```python
from build123d import *

# Parameters (mm, degrees)
F0_W            = 61.5
F0_H            = 60.53
F1_DEPTH        = 4.38
F3_DEPTH        = 31.34
F4_W            = 5.65
F4_H            = 8.3
F4_W_2          = 8.3
F4_H_2          = 5.65
F5_DEPTH        = 35.72
F7_DEPTH        = 35.72
F9_DEPTH        = 35.72
F11_D           = 3.5
F11_CSINK_D     = 10
F11_CSINK_ANGLE = 90
F13_D           = 3.5
F13_CSINK_D     = 10
F13_CSINK_ANGLE = 90
F15_D           = 3.5
F15_CSINK_D     = 10
F15_CSINK_ANGLE = 90
F17_D           = 3.5
F17_CSINK_D     = 10
F17_CSINK_ANGLE = 90


with BuildPart() as f1:
    # F0 (on Top) → F1 (new body)
    with BuildSketch(Plane.XY):
        with Locations((-10.297848, 8.882269)):
            Rectangle(F0_W, F0_H)
    extrude(amount=F1_DEPTH)

    # F2 (on face) → F3 (join)
    with BuildSketch(Plane.XY.offset(4.38)):
        Polygon((-41.047848, 39.147269), (-41.047848, -21.382731), (-35.397848, -21.382731), (-35.397848, 33.497269), (20.452152, 33.497269), (20.452152, 39.147269), (-35.397848, 39.147269), align=None)
    extrude(amount=F3_DEPTH)

    # F4 (on face) → F5 (cut, through all)
    with BuildSketch(Plane.XY.offset(35.72)):
        with Locations((-38.222848, -17.232731)):
            Rectangle(F4_W, F4_H)
        with Locations((16.302152, 36.322269)):
            Rectangle(F4_W_2, F4_H_2)
    extrude(amount=-F5_DEPTH, mode=Mode.SUBTRACT)

    # F6 (on face) → F7 (cut, through all)
    with BuildSketch(Plane.XY.offset(35.72)):
        Polygon((-41.047848, -13.082731), (-35.397848, -13.082731), (-41.047848, -7.432731), align=None)
        Polygon((6.502152, 39.147269), (12.152152, 33.497269), (12.152152, 39.147269), align=None)
    extrude(amount=-F7_DEPTH, mode=Mode.SUBTRACT)

    # F8 (on face) → F9 (cut, through all)
    with BuildSketch(Plane.XY.offset(35.72)):
        Polygon((-41.047848, 34.130973), (-36.031552, 39.147269), (-41.047848, 39.147269), align=None)
    extrude(amount=-F9_DEPTH, mode=Mode.SUBTRACT)

    # F11 (through all)
    with Locations(Plane.XY.offset(4.38)):
        with Locations((1.702152, -2.632731)):
            CounterSinkHole(F11_D / 2, F11_CSINK_D / 2, counter_sink_angle=F11_CSINK_ANGLE)

    # F13 (through all)
    with Locations(Plane.XY.offset(4.38)):
        with Locations((-20.897848, 19.967269)):
            CounterSinkHole(F13_D / 2, F13_CSINK_D / 2, counter_sink_angle=F13_CSINK_ANGLE)

    # F15 (through all)
    with Locations(Plane(origin=(0, 39.147269, 0), x_dir=(-1, 0, 0), z_dir=(0, 1, 0))):
        with Locations((13.497848, 22.12)):
            CounterSinkHole(F15_D / 2, F15_CSINK_D / 2, counter_sink_angle=F15_CSINK_ANGLE)

    # F17 (through all)
    with Locations(Plane(origin=(-41.047848, 0, 0), x_dir=(0, -1, 0), z_dir=(-1, 0, 0))):
        with Locations((-12.567269, 22.12)):
            CounterSinkHole(F17_D / 2, F17_CSINK_D / 2, counter_sink_angle=F17_CSINK_ANGLE)


solid = f1.part
```
Here's how the part is built. I have some questions about the finished solid (model axes, mm). A direction names the side the tool comes from. Give positions to 0.01 mm unless a question says otherwise; leave off trailing zeros. Write each loop counter-clockwise with the first axis right and the second up, starting at its lowest first coordinate (ties: lowest second). Pieces come first, ordered by that corner, then holes.
(1) Imagine slicing it at C-C, the plane y = -18. Write out the boundary of the cut face in (x, z).
Output values:
outline: (-35.4, 0) - (20.45, 0) - (20.45, 4.38) - (-35.4, 4.38) - close
(2) Thinking about a two-plate mould opening in X: for faces 1 (the face through (2.116, -4.495, 1.288)), 2 (the face through (-35.398, -17, 2)), 3 (the face through (9.29, 36.36, 18.11)), 4 (the face through (-36, 25, 35.72)), which applies, pulls with the +X half, pulls with the -X half, needs draft (parallel to the pull), parting line crosses it, or undercut?
Output values:
face 1: undercut
face 2: pulls with the -X half
face 3: pulls with the +X half
face 4: needs draft
(3) Will these pins go through, and if not, where does the flat tip stop? pin 1 (2 mm diameter, centred on x = -3.5, z = 9, fed in from -Y); pin 2 (3.5 mm diameter, centred on x = 15.5, z = 1.5, fed in from +Y); pin 3 (5 mm diameter, centred on y = -17, z = 2.5, fed in from -X).
Output values:
pin 1: stops at y = 33.5
pin 2: stops at y = 33.5
pin 3: stops at x = -35.4
(4) Imagine slicing it at B-B, the plane z = 9.5. Write out the boundary of the cut face in (x, y).
Output values:
outline: (-41.05, -7.43) - (-35.4, -13.08) - (-35.4, 33.5) - (12.15, 33.5) - (6.5, 39.15) - (-36.03, 39.15) - (-41.05, 34.13) - close
(5) On a 3-axis mill with a long thin cutter (end or side, diameter ignored), from which of +Z, -Z, +X, -X, +Y, -Y can I reach the whole of each face in a straight line? I mean faces 5 (the face through (-11, 9, 0)), 6 (the face through (-35.398, 10, 20)). Say none if no direction works.
Output values:
face 5: -Z, +X, -X, +Y, -Y
face 6: +Z, +X, -Y
(6) If I drill on L1, parallel to Y at x = -20, z = 21; L2, parallel to Z at x = 16, y = 22; L3, parallel to X at y = 15, z = 33, over which ranges is the centre line in solid material (lowest first)?
Output values:
L1: y = 33.5 to 39.15
L2: z = 0 to 4.38
L3: x = -41.05 to -35.4
(7) Imagine slicing it at D-D, the plane x = -33.5. Write out the boundary of the cut face in (y, z).
Output values:
outline: (-21.38, 0) - (39.15, 0) - (39.15, 35.72) - (33.5, 35.72) - (33.5, 4.38) - (-21.38, 4.38) - close
(8) Imagine slicing it at A-A, the plane z = 22.12. Write out the boundary of the cut face in (x, y).
Output values:
outline: (-41.05, -7.43) - (-35.4, -13.08) - (-35.4, 10.82) - (-37.8, 10.82) - (-41.05, 7.57) - close; (-41.05, 17.57) - (-37.8, 14.32) - (-35.4, 14.32) - (-35.4, 33.5) - (-15.25, 33.5) - (-15.25, 35.9) - (-18.5, 39.15) - (-36.03, 39.15) - (-41.05, 34.13) - close; (-11.75, 33.5) - (12.15, 33.5) - (6.5, 39.15) - (-8.5, 39.15) - (-11.75, 35.9) - close
